```python
from build123d import *

# Parameters (mm, degrees)
SKETCH_1_W          = 50.8
SKETCH_1_H          = 73.66
SKETCH_1_R          = 1.55
EXTRUDE_1_DEPTH     = 1.5
SKETCH_2_W          = 73.66
SKETCH_2_H          = 1.5
EXTRUDE_2_DEPTH     = 1.5
SKETCH_3_W          = 1.5
SKETCH_3_H          = 73.66
EXTRUDE_3_DEPTH     = 33.02
SKETCH_4_R          = 5.334
SKETCH_4_R_2        = 2.54
CUT_EXTRUDE_1_DEPTH = 33.02
SKETCH_6_W          = 1.5
SKETCH_6_H          = 73.66
EXTRUDE_4_DEPTH     = 1.5
SKETCH_7_W          = 73.66
SKETCH_7_H          = 1.5
EXTRUDE_5_DEPTH     = 31.98


with BuildPart() as part:
    # 草图1 → 凸台-拉伸1 (new body)
    with BuildSketch(Plane(origin=(0, 0, 0), x_dir=(1, 0, 0), z_dir=(0, 1, 0))):
        Rectangle(SKETCH_1_W, SKETCH_1_H)
        with Locations(Location((-22.86, 34.29, 0), (0, 0, 270))):
            Circle(SKETCH_1_R, mode=Mode.SUBTRACT)
        with Locations(Location((22.86, 34.29, 0), (0, 0, 270))):
            Circle(SKETCH_1_R, mode=Mode.SUBTRACT)
        with Locations(Location((22.86, -34.29, 0), (0, 0, 270))):
            Circle(SKETCH_1_R, mode=Mode.SUBTRACT)
        with Locations(Location((-22.86, -34.29, 0), (0, 0, 270))):
            Circle(SKETCH_1_R, mode=Mode.SUBTRACT)
    extrude(amount=EXTRUDE_1_DEPTH)

    # 草图2 → 凸台-拉伸2 (add)
    with BuildSketch(Plane.ZY.offset(25.4)):
        with Locations((0, 0.75)):
            Rectangle(SKETCH_2_W, SKETCH_2_H)
    extrude(amount=EXTRUDE_2_DEPTH)

    # 草图3 → 凸台-拉伸3 (add)
    with BuildSketch(Plane(origin=(0, 1.5, 0), x_dir=(1, 0, 0), z_dir=(0, 1, 0))):
        with Locations((-26.15, 0)):
            Rectangle(SKETCH_3_W, SKETCH_3_H)
    extrude(amount=EXTRUDE_3_DEPTH)

    # 草图4 → 切除-拉伸1 (cut)
    with BuildSketch(Plane(origin=(-25.4, 0, 0), x_dir=(0, 0, -1), z_dir=(1, 0, 0))):
        with Locations((0, 18.01)):
            Circle(SKETCH_4_R)
        with Locations((12.7, 18.01)):
            Circle(SKETCH_4_R_2)
        with Locations((25.4, 18.01)):
            Circle(SKETCH_4_R_2)
        with Locations((-12.7, 18.01)):
            Circle(SKETCH_4_R_2)
        with Locations((-25.4, 18.01)):
            Circle(SKETCH_4_R_2)
    extrude(amount=-CUT_EXTRUDE_1_DEPTH, mode=Mode.SUBTRACT)

    # 草图6 → 凸台-拉伸4 (add)
    with BuildSketch(Plane(origin=(0, 34.52, 0), x_dir=(1, 0, 0), z_dir=(0, 1, 0))):
        with Locations((-26.15, 0)):
            Rectangle(SKETCH_6_W, SKETCH_6_H)
    extrude(amount=EXTRUDE_4_DEPTH)

    # 草图7 → 凸台-拉伸5 (add)
    with BuildSketch(Plane(origin=(-25.4, 0, 0), x_dir=(0, 0, -1), z_dir=(1, 0, 0))):
        with Locations((0, 35.27)):
            Rectangle(SKETCH_7_W, SKETCH_7_H)
    extrude(amount=EXTRUDE_5_DEPTH)


solid = part.part
```
Work out the finished part from the listing and answer in its coordinate system (mm). A direction names the side the tool comes from. Coordinates: 2 decimals unless noted, no trailing zeros. Order: outer loops, then holes, each group sorted by start corner. A loop starts at its lowest first (then second) coordinate and runs counter-clockwise, first axis right, second up. Notation, with made-up numbers: (64.5, 31.25) - (89.5, 31.25) arc R25 cw to (89.5, 67.25) - close; hole circle Ø2 at (-29, -31). An arc over 180 degrees is marked (long way). Answer as a JSON object with one key per item and string values.
1. Find section C-C on x = 22.86. Determine the outline of the cut face in (y, z), plus the area to 3 significant figures.
Output values:
{"outline": "(0, -36.83) - (1.5, -36.83) - (1.5, -35.84) - (0, -35.84) - close; (0, -32.74) - (1.5, -32.74) - (1.5, 32.74) - (0, 32.74) - close; (0, 35.84) - (1.5, 35.84) - (1.5, 36.83) - (0, 36.83) - close", "area": "101 mm²"}
2. Find section A-A on x = -22.86. Determine the outline of the cut face in (y, z).
Output values:
{"outline": "(0, -36.83) - (1.5, -36.83) - (1.5, -35.84) - (0, -35.84) - close; (0, -32.74) - (1.5, -32.74) - (1.5, 32.74) - (0, 32.74) - close; (0, 35.84) - (1.5, 35.84) - (1.5, 36.83) - (0, 36.83) - close; (34.52, -36.83) - (36.02, -36.83) - (36.02, 36.83) - (34.52, 36.83) - close"}
3. Find section B-B on z = -34.29. Determine the outline of the cut face in (x, y).
Output values:
{"outline": "(-26.9, 0) - (-24.41, 0) - (-24.41, 1.5) - (-25.4, 1.5) - (-25.4, 34.52) - (6.58, 34.52) - (6.58, 36.02) - (-26.9, 36.02) - close; (-21.31, 0) - (21.31, 0) - (21.31, 1.5) - (-21.31, 1.5) - close; (24.41, 0) - (25.4, 0) - (25.4, 1.5) - (24.41, 1.5) - close"}
4. A tool of negligible diameter and unlimited length cuts with its end or side. For faces 5 (the face through (6.58, 35, 1)), 6 (the face through (-25.4, 10, 1)), 7 (the face through (-26.14, 16.464, 14.716)), 8 (the face through (-26, 15, -36.83)), 9 (the face through (-24.235, 0.74, 35.005)), from which of +Z, -Z, +X, -X, +Y, -Y can it reach the whole face along a straight path? Write none if from no direction.
Output values:
{"face 5": "+Z, -Z, +X, +Y", "face 6": "+Z, -Z, +X", "face 7": "+X, -X", "face 8": "-Z, +X, -X, +Y, -Y", "face 9": "-Y"}
5. Each of these flat-tipped pins is pushed along its axis until it touches: P1, Ø8, axis at y = 18.5, z = 19, coming from the +X side; P2, Ø5, axis at x = 22.86, z = 34.29, coming from the +Y side; P3, Ø8.5, axis at y = 18.01, z = 0, coming from the +X side. Where does it stop, or does it pass through?
Output values:
{"P1": "stops at x = -25.4", "P2": "stops at y = 1.5", "P3": "passes through"}
6. Consider line 1 (X direction, y = 0.4, z = -34.29); line 2 (Z direction, x = -26, y = 18); line 3 (Y direction, x = -14, z = 29). Determine where each line is inside the solid, lowest interval first.
Output values:
{"line 1": "x = -26.9 to -24.41, -21.31 to 21.31, 24.41 to 25.4", "line 2": "z = -36.83 to -27.94, -22.86 to -15.24, -10.16 to -5.33, 5.33 to 10.16, 15.24 to 22.86, 27.94 to 36.83", "line 3": "y = 0 to 1.5, 34.52 to 36.02"}
7. The mould has two halves that part along X. Classify faces 1 (the face through (-24.235, 0.74, -33.575)), 2 (the face through (-26.14, 18.122, 27.938)), 3 (the face through (22, 1, -33)), 4 (the face through (-26.9, 26, 1)): +X half, -X half, draft (parallel to the pull), parting line (faces both ways), or undercut.
Output values:
{"face 1": "undercut", "face 2": "draft", "face 3": "undercut", "face 4": "-X half"}
8. Find section D-D on z = -25.4. Determine the outline of the cut face in (x, y), plus the area to 3 significant figures.
Output values:
{"outline": "(-26.9, 0) - (25.4, 0) - (25.4, 1.5) - (-25.4, 1.5) - (-25.4, 15.47) - (-26.9, 15.47) - close; (-26.9, 20.55) - (-25.4, 20.55) - (-25.4, 34.52) - (6.58, 34.52) - (6.58, 36.02) - (-26.9, 36.02) - close", "area": "171 mm²"}
